from build123d import *

# Parameters (mm, degrees)
SKIZZE1_W                       = 35
SKIZZE1_H                       = 55.5
SKIZZE1_R                       = 16.1
SKIZZE1_R_2                     = 1.7
SKIZZE1_R_3                     = 2.3
AUFSATZ_LINEAR_AUSTRAGEN1_DEPTH = 11
SKIZZE2_W                       = 35
SKIZZE2_H                       = 35
SKIZZE2_R                       = 16.1
SKIZZE2_R_2                     = 1.7
AUFSATZ_LINEAR_AUSTRAGEN2_DEPTH = 19
SKIZZE4_R                       = 4
SCHNITT_LINEAR_AUSTRAGEN1_DEPTH = 8
SKIZZE5_R                       = 2.9
SCHNITT_LINEAR_AUSTRAGEN2_DEPTH = 27
FASE1_SIZE                      = 3
FASE2_SIZE                      = 8


with BuildPart() as part:
    # Skizze1 → Aufsatz-Linear austragen1 (new body)
    with BuildSketch(Plane.XY):
        with Locations((0, -10.25)):
            Rectangle(SKIZZE1_W, SKIZZE1_H)
        Circle(SKIZZE1_R, mode=Mode.SUBTRACT)
        with Locations((-13, 13)):
            Circle(SKIZZE1_R_2, mode=Mode.SUBTRACT)
        with Locations((13, 13)):
            Circle(SKIZZE1_R_2, mode=Mode.SUBTRACT)
        with Locations((-13, -13)):
            Circle(SKIZZE1_R_2, mode=Mode.SUBTRACT)
        with Locations((13, -13)):
            Circle(SKIZZE1_R_2, mode=Mode.SUBTRACT)
        with Locations((-12, -28)):
            Circle(SKIZZE1_R_3, mode=Mode.SUBTRACT)
        with Locations((12, -28)):
            Circle(SKIZZE1_R_3, mode=Mode.SUBTRACT)
    extrude(amount=AUFSATZ_LINEAR_AUSTRAGEN1_DEPTH)

    # Skizze2 → Aufsatz-Linear austragen2 (add)
    with BuildSketch(Plane.XY.offset(11)):
        Rectangle(SKIZZE2_W, SKIZZE2_H)
        Circle(SKIZZE2_R, mode=Mode.SUBTRACT)
        with Locations((13, 13)):
            Circle(SKIZZE2_R_2, mode=Mode.SUBTRACT)
        with Locations((13, -13)):
            Circle(SKIZZE2_R_2, mode=Mode.SUBTRACT)
        with Locations((-13, -13)):
            Circle(SKIZZE2_R_2, mode=Mode.SUBTRACT)
        with Locations((-13, 13)):
            Circle(SKIZZE2_R_2, mode=Mode.SUBTRACT)
    extrude(amount=AUFSATZ_LINEAR_AUSTRAGEN2_DEPTH)

    # Skizze4 → Schnitt-Linear austragen1 (cut)
    with BuildSketch(Plane.XY):
        with Locations((-12, -28)):
            Circle(SKIZZE4_R)
        with Locations((12, -28)):
            Circle(SKIZZE4_R)
    extrude(amount=SCHNITT_LINEAR_AUSTRAGEN1_DEPTH, mode=Mode.SUBTRACT)

    # Skizze5 → Schnitt-Linear austragen2 (cut)
    with BuildSketch(Plane.XY):
        with Locations((-13, 13)):
            Circle(SKIZZE5_R)
        with Locations((13, 13)):
            Circle(SKIZZE5_R)
        with Locations((-13, -13)):
            Circle(SKIZZE5_R)
        with Locations((13, -13)):
            Circle(SKIZZE5_R)
    extrude(amount=SCHNITT_LINEAR_AUSTRAGEN2_DEPTH, mode=Mode.SUBTRACT)

    # Fase1
    fase1_edges = [part.edges().sort_by_distance(p)[0] for p in [
        (-17.5, -17.5, 20.5),
        (17.5, -17.5, 20.5),
        (-17.5, 17.5, 15),
        (17.5, 17.5, 15),
    ]]
    chamfer(fase1_edges, length=FASE1_SIZE)

    # Fase2
    fase2_edges = [part.edges().sort_by_distance(p)[0] for p in [
        (17.5, -38, 5.5),
        (-17.5, -38, 5.5),
    ]]
    chamfer(fase2_edges, length=FASE2_SIZE)


solid = part.part
Design review of the part built by this model. Coordinates are the model's own, in mm. A direction names the side the tool comes from. Give positions to 0.01 mm unless a question says otherwise; leave off trailing zeros. Write each loop counter-clockwise with the first axis right and the second up, starting at its lowest first coordinate (ties: lowest second). Pieces come first, ordered by that corner, then holes. Notation, with made-up numbers: M -14,72 L -9,72 A25 ccw -9,92 Z; hole C 63.25,50.5 d3. An arc over 180 degrees is marked long. Answer as a JSON object with one key per item and string values. Group by question number.
1) We need section C-C (z = 9). Give the boundary of the cut face in (x, y), and give its area (3 significant figures).
2) Mouldability with a two-part tool opening along Y and no side actions: class faces 5 (the face through (-4, -16, 0)), 6 (the face through (-13.4, -34.1, 5.4)), 7 (the face through (14, -30, 8)), 8 (the face through (0, 17.5, 15)) as released by +Y, released by -Y, zero draft, split by the parting line, or undercut.
3) Tool access review of faces 1 (the face through (0, -17.5, 20)), 2 (the face through (-16, -16, 20)), 3 (the face through (13, -15, 27)), 4 (the face through (13.914, -11.567, 28.479)): name each direction out of +Z, -Z, +X, -X, +Y, -Y from which nothing blocks a thin tool from reaching the whole face with its end or side.
4) Clearance check with flat-ended pins moving along their axes: pin 1 Ø5.5 at (x, z) = (4.5, 19) entering from -Y; pin 2 Ø7 at (x, y) = (-4, -24.5) entering from +Z; pin 3 Ø3.5 at (x, y) = (-13, -13) entering from -Z. State where each tip first meets the part, or that it passes through.
5) For line 1 along Y through (x, z) = (-13, 18); line 2 along X through (y, z) = (-13, 28.8); line 3 along Y through (x, z) = (-13, 10), list the stretches that pass through material, from the lowest coordinate up.
6) We need section D-D (x = 7). Give the boundary of the cut face in (y, z), and give its area (3 significant figures).
7) We need section A-A (y = 0). Give the boundary of the cut face in (x, z).
8) We need section B-B (y = -28). Give the boundary of the cut face in (x, z), and give its area (3 significant figures).
Answer key:
{
 "1": {"outline": "M -17.5,-30 L -9.5,-38 L 9.5,-38 L 17.5,-30 L 17.5,14.5 L 14.5,17.5 L -14.5,17.5 L -17.5,14.5 Z; hole C -12,-28 d4.6; hole M -12.5,-10.14 A2.9 ccw long -10.14,-12.5 A16.1 ccw 10.14,-12.5 A2.9 ccw long 12.5,-10.14 A16.1 ccw 12.5,10.14 A2.9 ccw long 10.14,12.5 A16.1 ccw -10.14,12.5 A2.9 ccw long -12.5,10.14 A16.1 ccw Z; hole C 12,-28 d4.6", "area": "922 mm²"},
 "2": {"face 5": "zero draft", "face 6": "released by -Y", "face 7": "undercut", "face 8": "released by +Y"},
 "3": {"face 1": "+Z, +X, -X, -Y", "face 2": "+Z, -X, -Y", "face 3": "-Z", "face 4": "+Z, -Z"},
 "4": {"pin 1": "stops at y = -17.5", "pin 2": "stops at z = 11", "pin 3": "stops at z = 27"},
 "5": {"line 1": "y = -17.5 to -15.9, -10.1 to -9.5, 9.5 to 10.1, 15.9 to 17.5", "line 2": "x = -17.5 to -14.7, -11.3 to -9.5, 9.5 to 11.3, 14.7 to 17.5", "line 3": "y = -34.5 to -30.07, -25.93 to -15.9, -10.1 to -9.5, 9.5 to 10.1, 15.9 to 17.5"},
 "6": {"outline": "M -38,0 L -14.5,0 L -14.5,30 L -17.5,30 L -17.5,11 L -38,11 Z; M 14.5,0 L 17.5,0 L 17.5,30 L 14.5,30 Z", "area": "406 mm²"},
 "7": {"outline": "M -17.5,0 L -16.1,0 L -16.1,30 L -17.5,30 Z; M 16.1,0 L 17.5,0 L 17.5,30 L 16.1,30 Z"},
 "8": {"outline": "M -17.5,0 L -16,0 L -16,8 L -14.3,8 L -14.3,11 L -17.5,11 Z; M -9.7,8 L -8,8 L -8,0 L 8,0 L 8,8 L 9.7,8 L 9.7,11 L -9.7,11 Z; M 14.3,8 L 16,8 L 16,0 L 17.5,0 L 17.5,11 L 14.3,11 Z", "area": "229 mm²"}
}
